For this review, take the finished solid that the model builds, in its own axes (mm). A direction names the side the tool comes from. Give positions to 0.01 mm unless a question says otherwise; leave off trailing zeros. Order: outer loops, then holes, each group sorted by start corner. A loop starts at its lowest first (then second) coordinate and runs counter-clockwise, first axis right, second up. Notation, with made-up numbers: (75.5, 33.25) -> (101.5, 33.25) arc R15 ccw to (101.5, 45.25) -> close; hole circle Ø9 at (56, 9.5). An arc over 180 degrees is marked (long way). Return JSON: item names as keys, results as strings. Group by question number.
1) To check wall thickness, follow line 1 along Y through (x, z) = (29, 4.5); line 2 along Y through (x, z) = (-29, 8.75); line 3 along Y through (x, z) = (-69, 3.5). State the ranges of each line that lie inside material, in increasing order.
2) Add section B-B (z = 7). State how many separate pieces and enclosed holes the cut face has, then the cut area to 3 significant figures.
3) Add section A-A (x = -5.5). Give the boundary of the cut face in (y, z) (3 decimals).
4) The part is to be moulded in two halves that separate along Y. For faces 4 (the face through (72, 10.319, 5)), 5 (the face through (76.2, 23, 5)), 6 (the face through (-19.823, 18.37, 4.696)), 7 (the face through (1, 35.719, 5)), say which applies: released by +Y, released by -Y, zero draft, split by the parting line, or undercut.
5) For faces 1 (the face through (-76.2, 23, 5)), 2 (the face through (-72, 10.319, 5)), 3 (the face through (0.734, 28.313, 4.696)), list the 3-axis set-ups (+Z, -Z, +X, -X, +Y, -Y) from which the entire face can be reached by the end or side of a thin tool; tool diameter is ignored.
6) Insertion check: P1, Ø5, axis at x = 2.5, z = 1.5, coming from the -Y side. The pin has a flat end and moves straight along its axis. Give the tip position at first contact, or say it passes through.
from build123d import *

# Parameters (mm, degrees)
F0_R     = 2.5796875
F1_DEPTH = 9.525


with BuildPart() as f1:
    # F0 (on Top) → F1 (new body)
    with BuildSketch(Plane.XY):
        with BuildLine():
            Line((76.2, 35.71875), (0, 35.71875))
            Line((0, 35.71875), (-76.2, 35.71875))
            Line((-76.2, 35.71875), (-76.2, 10.31875))
            Line((-76.2, 10.31875), (-67.3197399736, 10.31875))
            add(Edge.make_bspline(
                [(-67.3197399736, 10.31875), (-61.8867674924, 10.2547754123), (-47.5386632194, 6.8807184355), (-34.2599964973, 0), (-28.575, 0)],
                knots=[0, 0, 0, 0, 0.4984157806, 1, 1, 1, 1], degree=3))
            Line((-28.575, 0), (0, 0))
            Line((0, 0), (28.575, 0))
            add(Edge.make_bspline(
                [(67.3197399736, 10.31875), (61.8867674924, 10.2547754123), (47.5386632194, 6.8807184355), (34.2599964973, 0), (28.575, 0)],
                knots=[0, 0, 0, 0, 0.4984157806, 1, 1, 1, 1], degree=3))
            Line((67.3197399736, 10.31875), (76.2, 10.31875))
            Line((76.2, 10.31875), (76.2, 35.71875))
        make_face()
        with Locations((-29.6867411598, 18.25625)):
            Circle(F0_R, mode=Mode.SUBTRACT)
        with Locations((-17.2455671598, 18.25625)):
            Circle(F0_R, mode=Mode.SUBTRACT)
        with Locations((-5.0710931598, 18.25625)):
            Circle(F0_R, mode=Mode.SUBTRACT)
        with Locations((6.8747808402, 18.25625)):
            Circle(F0_R, mode=Mode.SUBTRACT)
        with Locations((18.6174548402, 18.25625)):
            Circle(F0_R, mode=Mode.SUBTRACT)
        with Locations((30.2077288402, 18.25625)):
            Circle(F0_R, mode=Mode.SUBTRACT)
        with BuildLine():
            ThreePointArc((-29.6326200987, 26.9315806998), (-30.87613546, 28.0668539389), (-29.7408622209, 29.3103693002))
            Line((-29.7408622209, 29.3103693002), (30.1536077791, 32.03575))
            ThreePointArc((30.1536077791, 32.03575), (31.3971231404, 30.9004767609), (30.2618499013, 29.6569613996))
            Line((30.2618499013, 29.6569613996), (-29.6326200987, 26.9315806998))
        make_face(mode=Mode.SUBTRACT)
    extrude(amount=F1_DEPTH)


solid = f1.part
Evaluation:
{
 "1": {"line 1": "0.01 to 15.98, 20.54 to 29.6, 31.98 to 35.72", "line 2": "0.01 to 15.77, 20.74 to 26.96, 29.34 to 35.72", "line 3": "10.32 to 35.72"},
 "2": {"separate pieces": "1", "enclosed holes": "7", "area": "4,550 mm^2"},
 "3": {"outline": "(0, 0) -> (15.712, 0) -> (15.712, 9.525) -> (0, 9.525) -> close; (20.8, 0) -> (28.03, 0) -> (28.03, 9.525) -> (20.8, 9.525) -> close; (30.413, 0) -> (35.719, 0) -> (35.719, 9.525) -> (30.413, 9.525) -> close"},
 "4": {"face 4": "released by -Y", "face 5": "zero draft", "face 6": "undercut", "face 7": "released by +Y"},
 "5": {"face 1": "+Z, -Z, -X, +Y, -Y", "face 2": "+Z, -Z, -X, -Y", "face 3": "+Z, -Z"},
 "6": {"P1": "y = 0"}
}
